from build123d import *

# Parameters (mm, degrees)
SKETCH_1_R      = 1.25
EXTRUDE_1_DEPTH = 17.5


with BuildPart() as part:
    # 草图1 → 凸台-拉伸1 (new body)
    with BuildSketch(Plane(origin=(0, 0, 0), x_dir=(1, 0, 0), z_dir=(0, 1, 0))):
        with BuildLine():
            Line((-40.9, 0), (-40.9, 46.9))
            Line((-40.9, 46.9), (-42.9, 46.9))
            Line((-42.9, 46.9), (-42.9, 44.02953021))
            ThreePointArc((-42.9, 44.02953021), (-43.350806662, 42.764619146), (-44.5, 42.069938416))
            ThreePointArc((-44.5, 42.069938416), (-46.9, 39.130550724), (-44.5, 36.191163033))
            ThreePointArc((-44.5, 36.191163033), (-43.350806662, 35.496482303), (-42.9, 34.231571239))
            Line((-42.9, 34.231571239), (-42.9, 4.898979486))
            ThreePointArc((-42.9, 4.898979486), (-43.350806662, 3.634068421), (-44.5, 2.939387691))
            ThreePointArc((-44.5, 2.939387691), (-46.898844518, -0.083255983), (-44.335990888, -2.968149583))
            ThreePointArc((-44.335990888, -2.968149583), (-43.187596963, -3.557987573), (-42.638827361, -4.726563367))
            ThreePointArc((-42.638827361, -4.726563367), (-30.334880913, -30.334880913), (-4.726563367, -42.638827361))
            ThreePointArc((-4.726563367, -42.638827361), (-3.557987573, -43.187596963), (-2.968149583, -44.335990888))
            ThreePointArc((-2.968149583, -44.335990888), (0, -46.9), (2.968149583, -44.335990888))
            ThreePointArc((2.968149583, -44.335990888), (3.557987573, -43.187596963), (4.726563367, -42.638827361))
            ThreePointArc((4.726563367, -42.638827361), (30.334880913, -30.334880913), (42.638827361, -4.726563367))
            ThreePointArc((42.638827361, -4.726563367), (43.187596963, -3.557987573), (44.335990888, -2.968149583))
            ThreePointArc((44.335990888, -2.968149583), (46.9, 0), (44.335990888, 2.968149583))
            ThreePointArc((44.335990888, 2.968149583), (43.187596963, 3.557987573), (42.638827361, 4.726563367))
            ThreePointArc((42.638827361, 4.726563367), (30.334880913, 30.334880913), (4.726563367, 42.638827361))
            ThreePointArc((4.726563367, 42.638827361), (3.557987573, 43.187596963), (2.968149583, 44.335990888))
            ThreePointArc((2.968149583, 44.335990888), (0, 46.9), (-2.968149583, 44.335990888))
            ThreePointArc((-2.968149583, 44.335990888), (-3.557987573, 43.187596963), (-4.726563367, 42.638827361))
            ThreePointArc((-4.726563367, 42.638827361), (-9.998714121, 41.718529647), (-15.115253688, 40.148961455))
            ThreePointArc((-15.115253688, 40.148961455), (-16.405630214, 40.108391944), (-17.451956512, 40.864645036))
            ThreePointArc((-17.451956512, 40.864645036), (-18.261151224, 41.643352884), (-19.3, 42.069938416))
            ThreePointArc((-19.3, 42.069938416), (-20.449193338, 42.764619146), (-20.9, 44.02953021))
            Line((-20.9, 44.02953021), (-20.9, 46.9))
            Line((-20.9, 46.9), (-22.9, 46.9))
            Line((-22.9, 46.9), (-22.9, 33.888050991))
            ThreePointArc((-22.9, 33.888050991), (36.120769649, -19.185932346), (-40.9, 0))
        make_face()
        with Locations((0, 43.9)):
            Circle(SKETCH_1_R, mode=Mode.SUBTRACT)
        with Locations((43.9, 0)):
            Circle(SKETCH_1_R, mode=Mode.SUBTRACT)
        with Locations((0, -43.9)):
            Circle(SKETCH_1_R, mode=Mode.SUBTRACT)
        with Locations((-43.9, 0)):
            Circle(SKETCH_1_R, mode=Mode.SUBTRACT)
        with Locations((-19.9, 39.130550724)):
            Circle(SKETCH_1_R, mode=Mode.SUBTRACT)
        with Locations((-43.9, 39.130550724)):
            Circle(SKETCH_1_R, mode=Mode.SUBTRACT)
    extrude(amount=EXTRUDE_1_DEPTH)


solid = part.part
The listing builds one solid part. Answer for the finished solid, in the listing's coordinates (mm). A direction names the side the tool comes from. Round coordinates to 2 decimals unless told otherwise and drop trailing zeros. Write each loop counter-clockwise with the first axis right and the second up, starting at its lowest first coordinate (ties: lowest second). Pieces come first, ordered by that corner, then holes. Notation, with made-up numbers: (15, 33) - (71, 33) arc R24 cw to (71, 58) - close; hole circle Ø10 at (-18, 63). An arc over 180 degrees is marked (long way). Use a Markdown table: item, result. Add a question column.
1. The part is cut by section A-A (x = 0). Write down the section's boundary in (y, z).
2. A tool of negligible diameter and unlimited length cuts with its end or side. For faces 1 (the face through (-40.9, 9, -23)), 2 (the face through (-30.62, 8.628, 30.047)), 3 (the face through (-42.9, 9, -45)), from which of +Z, -Z, +X, -X, +Y, -Y can it reach the whole face along a straight path? Write none if from no direction.
3. Flat-ended cylindrical pins translate along their axes: P1, Ø2, axis at x = -43.9, z = 0, coming from the +Y side; P2, Ø4, axis at y = 2, z = 0.5, coming from the -X side; P3, Ø2, axis at y = 11.5, z = 18, coming from the -X side; P4, Ø2, axis at y = 11, z = 21.5, coming from the +X side (3 decimals). Find the tip coordinate at first contact, or state that the pin passes through.
4. For a pull along Z with two mould halves and no side action, classify faces 4 (the face through (30.047, 8.628, 30.62)), 5 (the face through (-22.9, 9, -40)), 6 (the face through (-0.16, 8.63, -45.14)) as +Z half, -Z half, draft (parallel to the pull), parting line (faces both ways), or undercut.
5. The part is cut by section D-D (y = 13.75). Give the number of separate pieces and of enclosed holes in the cut face, and give its area (3 significant figures).
6. Consider line 1 (Z direction, x = 0, y = 12.25); line 2 (Z direction, x = -43.9, y = 11.5); line 3 (Z direction, x = -19.9, y = 7.5). Determine where each line is inside the solid, lowest interval first.
7. The part is cut by section C-C (x = 38.5). Write down the section's boundary in (y, z), and give its area (3 significant figures).
8. The part is cut by section B-B (z = 11.5). Write down the section's boundary in (x, y).
Reported:
| question | item | result |
|---|---|---|
| 1 | outline | (0, -46.9) - (17.5, -46.9) - (17.5, -45.15) - (0, -45.15) - close; (0, -42.65) - (17.5, -42.65) - (17.5, -40.9) - (0, -40.9) - close; (0, 40.9) - (17.5, 40.9) - (17.5, 42.65) - (0, 42.65) - close; (0, 45.15) - (17.5, 45.15) - (17.5, 46.9) - (0, 46.9) - close |
| 2 | face 1 | -Z, +Y, -Y |
| 2 | face 2 | +Z, -X, +Y, -Y |
| 2 | face 3 | -Z, -X, +Y, -Y |
| 3 | P1 | through |
| 3 | P2 | x = -46.9 |
| 3 | P3 | x = -39.39 |
| 3 | P4 | x = 37.685 |
| 4 | face 4 | +Z half |
| 4 | face 5 | draft |
| 4 | face 6 | undercut |
| 5 | separate pieces | 1 |
| 5 | enclosed holes | 6 |
| 5 | area | 650 mm^2 |
| 6 | line 1 | -46.9 to -45.15, -42.65 to -40.9, 40.9 to 42.65, 45.15 to 46.9 |
| 6 | line 2 | -42.3 to -40.38, -37.88 to -35.96, -3.17 to -1.25, 1.25 to 3.08 |
| 6 | line 3 | -42.3 to -40.38, -37.88 to -35.73, 35.73 to 38.01 |
| 7 | outline | (0, -18.93) - (17.5, -18.93) - (17.5, -13.8) - (0, -13.8) - close; (0, 13.8) - (17.5, 13.8) - (17.5, 18.93) - (0, 18.93) - close |
| 7 | area | 179 mm^2 |
| 8 | outline | (-41.33, 0) - (-39.25, 0) - (-39.25, 17.5) - (-41.33, 17.5) - close; (39.25, 0) - (41.33, 0) - (41.33, 17.5) - (39.25, 17.5) - close |
